The model under review builds one solid part; all positions refer to its coordinate system, in mm. Face numbers are marked on the shaded views. A direction names the side the tool comes from. Round coordinates to 2 decimals unless told otherwise and drop trailing zeros. Order: outer loops, then holes, each group sorted by start corner. A loop starts at its lowest first (then second) coordinate and runs counter-clockwise, first axis right, second up. Notation, with made-up numbers: (-20.5, 40.25) - (26.5, 40.25) arc R9 cw to (26.5, 47.25) - close; hole circle Ø10 at (11.25, -6.75). An arc over 180 degrees is marked (long way). One line per question, with ' | ' between items. Start each with the question number.
Item 1: Insertion check: pin 1 Ø6 at (x, z) = (-2.5, 14) entering from -Y; pin 2 Ø1.5 at (x, z) = (0, 32) entering from -Y; pin 3 Ø12 at (x, y) = (-7, -1.5) entering from -Z. Each pin has a flat end and moves straight along its axis. Give the tip position at first contact, or say it passes through.
Item 2: Add section D-D on y = 9.5. State the section outline as (x, z) points, and give its area (3 significant figures).
Item 3: Tool access review of the marked faces 1, 2, 3 and 4: name each direction out of +Z, -Z, +X, -X, +Y, -Y from which nothing blocks a thin tool from reaching the whole face with its end or side.
Item 4: For L1, parallel to Z at x = 0.25, y = -6.5; L2, parallel to X at y = -14.75, z = -4; L3, parallel to Z at x = -4.25, y = -13.75, list the stretches that pass through material, from the lowest coordinate up. Write a range as [from, to].
Item 5: Add section C-C on z = 16. State the section outline as (x, y) points.
Item 6: Draft analysis for pull direction Z (two halves, no side actions). For the marked faces 5, 6 and 7, state which applies: +Z half, -Z half, draft (parallel to the pull), parting line (faces both ways), or undercut.
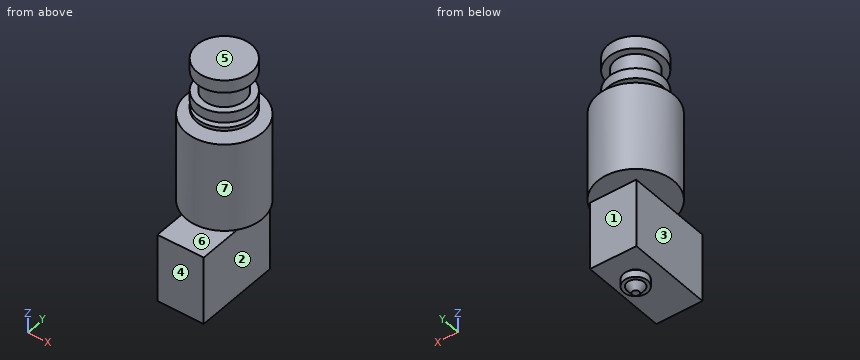
from build123d import *

# Parameters (mm, degrees)
F2_R     = 2.5
F3_DEPTH = 3
F4_W     = 13.5
F4_H     = 25
F5_DEPTH = 20


with BuildPart() as f1:
    # F0 (on Front) → F1 (revolve)
    with BuildSketch(Plane.XZ):
        Polygon((0, 42.7), (0, 0), (11.15, 0), (11.15, 26), (6, 26), (6, 27.5), (8, 27.5), (8, 28.5), (6, 28.5), (6, 30), (8, 30), (8, 33), (6, 33), (6, 39), (8, 39), (8, 42.7), align=None)
    revolve(axis=Axis((0, 0, 21.35), (0, 0, 1)))

    # F2 (on face) → F3 (join)
    with BuildSketch(Plane(origin=(0, 0, 0), x_dir=(1, 0, 0), z_dir=(0, 0, -1))):
        Circle(F2_R)
    extrude(amount=F3_DEPTH)

    # F4 (on face) → F5 (join)
    with BuildSketch(Plane(origin=(0, 0, -3), x_dir=(1, 0, 0), z_dir=(0, 0, -1))):
        with Locations((0, 4)):
            Rectangle(F4_W, F4_H)
    extrude(amount=F5_DEPTH)

    # F6 (on Front) → F7 (revolve)
    with BuildSketch(Plane.XZ):
        Polygon((0, -28.1), (0, -23), (-2.5, -23), (-2.5, -24), (-3.5, -24), (-3.5, -26.1), (-2.5, -26.1), (-1, -28.1), align=None)
    revolve(axis=Axis((0, 0, -25.55), (0, 0, -1)))


solid = f1.part
Determined:
1) pin 1: y = -11.15 | pin 2: y = -8 | pin 3: z = -27.89
2) outline: (-5.84, 0) - (5.84, 0) - (5.84, 26) - (-5.84, 26) - close | area: 304 mm2
3) face 1: -Z, +X, -X, +Y | face 2: -Z, +X, +Y, -Y | face 3: -Z, -X, +Y, -Y | face 4: +Z, -Z, +X, -X, -Y
4) L1: [-23, -3], [0, 26], [27.5, 28.5], [30, 33], [39, 42.7] | L2: [-6.75, 6.75] | L3: [-23, -3]
5) outline: circle Ø22.3 at (0, 0)
6) face 5: +Z half | face 6: undercut | face 7: draft
